```python
from build123d import *

# Parameters (mm, degrees)
EXTRUDE_1_DEPTH     = 15
SKETCH_2_R          = 3.4
CUT_EXTRUDE_2_DEPTH = 1193.231762859
SKETCH_3_R          = 5
CUT_EXTRUDE_3_DEPTH = 14


with BuildPart() as part:
    # 草图1 → 拉伸1 (new body)
    with BuildSketch(Plane.XY):
        with BuildLine():
            Line((1175.612511144, 1087.358821907), (1190.725651177, 1087.358821907))
            Line((1190.725651177, 1087.358821907), (1190.725651177, 1100.858821907))
            Line((1190.725651177, 1100.858821907), (1160.725651177, 1100.858821907))
            ThreePointArc((1160.725651177, 1100.858821907), (1153.654583365, 1097.929889719), (1150.725651177, 1090.858821907))
            Line((1150.725651177, 1090.858821907), (1150.725651177, 1072.358821907))
            ThreePointArc((1150.725651177, 1072.358821907), (1151.018544396, 1071.651715126), (1151.725651177, 1071.358821907))
            Line((1151.725651177, 1071.358821907), (1152.725651177, 1071.358821907))
            ThreePointArc((1152.725651177, 1071.358821907), (1156.261185083, 1069.894355813), (1157.725651177, 1066.358821907))
            Line((1157.725651177, 1066.358821907), (1157.725651177, 1050.858821907))
            ThreePointArc((1157.725651177, 1050.858821907), (1165.725651177, 1042.858821907), (1173.725651177, 1050.858821907))
            Line((1173.725651177, 1050.858821907), (1173.725651177, 1066.358821907))
            ThreePointArc((1173.725651177, 1066.358821907), (1175.190117271, 1069.894355813), (1178.725651177, 1071.358821907))
            Line((1178.725651177, 1071.358821907), (1190.725651177, 1071.358821907))
            Line((1190.725651177, 1071.358821907), (1190.725651177, 1084.358821907))
            Line((1190.725651177, 1084.358821907), (1175.612511144, 1084.358821907))
            ThreePointArc((1175.612511144, 1084.358821907), (1175.056800803, 1082.26304012), (1174.062422361, 1080.336300179))
            ThreePointArc((1174.062422361, 1080.336300179), (1174.210932551, 1077.373540533), (1171.248172905, 1077.522050723))
            ThreePointArc((1171.248172905, 1077.522050723), (1165.725651177, 1075.858821907), (1160.203129449, 1077.522050723))
            ThreePointArc((1160.203129449, 1077.522050723), (1157.240369803, 1077.373540533), (1157.388879993, 1080.336300179))
            ThreePointArc((1157.388879993, 1080.336300179), (1155.725651177, 1085.858821907), (1157.388879993, 1091.381343635))
            ThreePointArc((1157.388879993, 1091.381343635), (1157.240369803, 1094.344103281), (1160.203129449, 1094.195593091))
            ThreePointArc((1160.203129449, 1094.195593091), (1165.725651177, 1095.858821907), (1171.248172905, 1094.195593091))
            ThreePointArc((1171.248172905, 1094.195593091), (1174.210932551, 1094.344103281), (1174.062422361, 1091.381343635))
            ThreePointArc((1174.062422361, 1091.381343635), (1175.056800803, 1089.454603694), (1175.612511144, 1087.358821907))
        make_face()
    extrude(amount=EXTRUDE_1_DEPTH)

    # 草图2 → 拉伸2 (cut, through all)
    with BuildSketch(Plane(origin=(0, 1100.858821907, 0), x_dir=(1, 0, 0), z_dir=(0, 1, 0))):
        with Locations((1182.725651177, -7.5)):
            Circle(SKETCH_2_R)
    extrude(amount=-CUT_EXTRUDE_2_DEPTH, mode=Mode.SUBTRACT)

    # 草图3 → 拉伸3 (cut)
    with BuildSketch(Plane(origin=(0, 1100.858821907, 0), x_dir=(1, 0, 0), z_dir=(0, 1, 0))):
        with Locations(Location((1182.725651177, -7.5, 0), (0, 0, 270))):
            Circle(SKETCH_3_R)
    extrude(amount=-CUT_EXTRUDE_3_DEPTH, mode=Mode.SUBTRACT)


solid = part.part
```
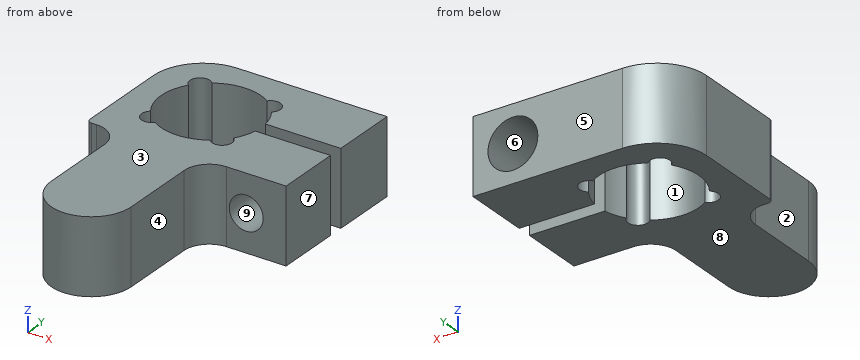
For this review, take the finished solid that the model builds, in its own axes (mm). Face numbers are marked on the shaded views. A direction names the side the tool comes from. Coordinates: 2 decimals unless noted, no trailing zeros. Write each loop counter-clockwise with the first axis right and the second up, starting at its lowest first coordinate (ties: lowest second). Pieces come first, ordered by that corner, then holes. Notation, with made-up numbers: (61, 25) - (97, 25) arc R10 cw to (97, 40) - close; hole circle Ø10 at (-31, 6.5). An arc over 180 degrees is marked (long way). Put each result on its own line as item: value.
1. Mouldability with a two-part tool opening along Z and no side actions: class the marked faces 6, 7, 8 and 9 as released by +Z, released by -Z, zero draft, split by the parting line, or undercut.
Values found:
face 6: undercut
face 7: zero draft
face 8: released by -Z
face 9: undercut
2. Machinability: for the marked faces 1, 2, 3, 4 and 5, which of the approach directions +Z, -Z, +X, -X, +Y, -Y give a long, thin tool a straight path to every point of the face, cutting with its end or side? Answer none if there is none.
Values found:
face 1: +Z, -Z
face 2: +Z, -Z, -X, -Y
face 3: +Z, +X, -X, +Y, -Y
face 4: +Z, -Z, +X, -Y
face 5: +Z, -Z, +X, -X, +Y
3. Add section C-C, the plane z = 7.5. Count the separate pieces of the cut face and the enclosed holes in it, then the cut area to 3 significant figures.
Values found:
separate pieces: 3
enclosed holes: 0
area: 989 mm²
4. Add section B-B, the plane x = 1185.5. Give the boundary of the cut face in (y, z), then the cut area to 3 significant figures.
Values found:
outline: (1071.36, 0) - (1084.36, 0) - (1084.36, 5.53) - (1071.36, 5.53) - close; (1071.36, 9.47) - (1084.36, 9.47) - (1084.36, 15) - (1071.36, 15) - close; (1087.36, 0) - (1100.86, 0) - (1100.86, 3.34) - (1087.36, 3.34) - close; (1087.36, 11.66) - (1100.86, 11.66) - (1100.86, 15) - (1087.36, 15) - close
area: 234 mm²
5. For pin 1 (3.5 mm diameter, centred on x = 1186.5, z = 5.5, fed in from -Y); pin 2 (4.5 mm diameter, centred on y = 1059.5, z = 8, fed in from -X); pin 3 (1 mm diameter, centred on y = 1063.5, z = 9, fed in from +X), all flat-tipped, find the tip position at first contact; note any pin that passes through.
Values found:
pin 1: y = 1071.36
pin 2: x = 1157.73
pin 3: x = 1173.73
6. Wall thickness on probe 1 along Y at (x, z) = (1174.5, 12); probe 2 along Y at (x, z) = (1186.5, 3.5); probe 3 along X at (y, z) = (1080, 4.75): over which ranges is each line inside the solid? List them lowest first.
Values found:
probe 1: 1069.03 to 1077.74, 1079.84 to 1081.06, 1090.66 to 1091.88, 1093.98 to 1100.86
probe 2: 1071.36 to 1084.36, 1087.36 to 1100.86
probe 3: 1150.73 to 1157.06, 1174.39 to 1180.73, 1184.73 to 1190.73
7. Add section D-D, the plane x = 1166.5. Give the boundary of the cut face in (y, z), then the cut area to 3 significant figures.
Values found:
outline: (1042.9, 0) - (1075.89, 0) - (1075.89, 15) - (1042.9, 15) - close; (1095.83, 0) - (1100.86, 0) - (1100.86, 15) - (1095.83, 15) - close
area: 570 mm²
8. Add section A-A, the plane y = 1079.5. Give the boundary of the cut face in (x, z).
Values found:
outline: (1150.73, 0) - (1156.79, 0) - (1156.79, 15) - (1150.73, 15) - close; (1174.67, 0) - (1190.73, 0) - (1190.73, 15) - (1174.67, 15) - close; hole circle Ø6.8 at (1182.73, 7.5)
